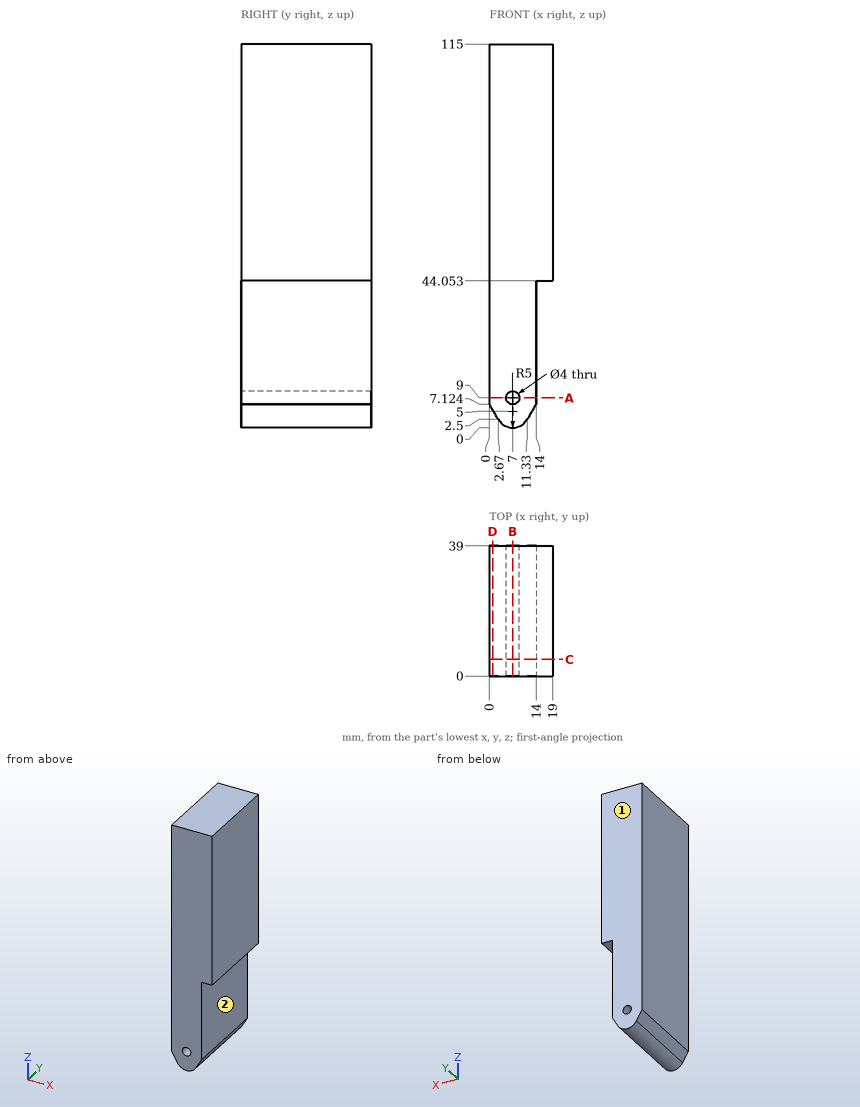
Job drawing, mm, ordinate dimensions from the low corner. One solid piece. A direction names the side the tool comes from. Round coordinates to 2 decimals unless told otherwise and drop trailing zeros. Write each loop counter-clockwise with the first axis right and the second up, starting at its lowest first coordinate (ties: lowest second). Pieces come first, ordered by that corner, then holes. Notation, with made-up numbers: M -21,22.5 L 25,22.5 A17 ccw 25,44.5 Z; hole C 48,53.25 d4. An arc over 180 degrees is marked long. Return JSON: item names as keys, results as strings. Group by question number.
(1) Pin check, flat tips, straight feed: pin 1 Ø4 at (x, y) = (10, 11) entering from -Z; pin 2 Ø4 at (x, y) = (11.5, 19.5) entering from -Z; pin 3 Ø4 at (x, y) = (16.5, 17) entering from -Z. Stop position of each tip, or through.
(2) Saw through at A-A on z = 9. Write the cut outline in (x, y), then the cut area to 3 significant figures.
(3) Drill centre lines: probe 1 along X at (y, z) = (19, 9); probe 2 along Z at (x, y) = (15, 32.5); probe 3 along X at (y, z) = (31, 30). Where is each one in solid material? Low to high.
(4) Saw through at C-C on y = 5. Write the cut outline in (x, z) (1 decimal), then the cut area to 3 significant figures.
(5) Saw through at B-B on x = 7. Write the cut outline in (y, z), then the cut area to 3 significant figures.
(6) Saw through at D-D on x = 1. Write the cut outline in (y, z), then the cut area to 3 significant figures.
(7) Which spindle directions (+Z, -Z, +X, -X, +Y, -Y) get a long thin tool onto all of the face, cutting with end or side? Do the marked faces 1 and 2. Say none if no direction does.
Returned:
{
 "1": {"pin 1": "z = 0.1", "pin 2": "z = 0.67", "pin 3": "z = 44.05"},
 "2": {"outline": "M 0,0 L 5,0 L 5,39 L 0,39 Z; M 9,0 L 14,0 L 14,39 L 9,39 Z", "area": "390 mm²"},
 "3": {"probe 1": "0 to 5, 9 to 14", "probe 2": "44.05 to 115", "probe 3": "0 to 14"},
 "4": {"outline": "M 0,7.1 L 2.7,2.5 A5 ccw 11.3,2.5 L 14,7.1 L 14,44.1 L 19,44.1 L 19,115 L 0,115 Z; hole C 7,9 d4", "area": "1,920 mm²"},
 "5": {"outline": "M 0,0 L 39,0 L 39,7 L 0,7 Z; M 0,11 L 39,11 L 39,115 L 0,115 Z", "area": "4,330 mm²"},
 "6": {"outline": "M 0,5.39 L 39,5.39 L 39,115 L 0,115 Z", "area": "4,270 mm²"},
 "7": {"face 1": "+Z, -Z, +X, -X, +Y", "face 2": "-Z, +X, +Y, -Y"}
}
